Source: CAD feature listing. Evaluate the final solid. Frame: model axes, mm. Round coordinates to 2 decimals unless told otherwise and drop trailing zeros. Loops run counter-clockwise (first coordinate to the right, second up) from the corner with the lowest first, then second, coordinate; pieces in that order, holes last. Notation, with made-up numbers: (-37, 82.5) - (7, 82.5) arc R30 cw to (7, 113.5) - close; hole circle Ø1 at (29.25, 41.25). An arc over 180 degrees is marked (long way). One line per question, with ' | ' between items.
from build123d import *

# Parameters (mm, degrees)
BOSS_EXTRUDE1_DEPTH         = 6.35
FILLET1_R                   = 101.6
F_1_4_CLEARANCE_SLOT1_DEPTH = 6.35
FILLET2_R                   = 6.35


# Read off the part's stored shape, not the designer's step: 1/4 Clearance Slot1
with BuildPart() as part:
    # Sketch1 → Boss-Extrude1 (new body)
    with BuildSketch(Plane(origin=(0, 0, 0), x_dir=(0, 0, -1), z_dir=(1, 0, 0))):
        Polygon((0, 0), (0, 152.4), (654.05, 152.4), (717.55, 38.1), (717.55, 0), align=None)
    extrude(amount=BOSS_EXTRUDE1_DEPTH)

    # Fillet1
    fillet1_edges = [part.edges().sort_by_distance(p)[0] for p in [
        (3.175, 152.4, -654.05),
    ]]
    fillet(fillet1_edges, radius=FILLET1_R)

    # 1/4 Clearance Slot1 outline → 1/4 Clearance Slot1 (cut)
    with BuildSketch(Plane.YZ):
        with BuildLine():
            ThreePointArc((25.6032, -698.7032), (22.225, -695.325), (18.8468, -698.7032))
            Line((18.8468, -698.7032), (18.8468, -704.6468))
            ThreePointArc((18.8468, -704.6468), (22.225, -708.025), (25.6032, -704.6468))
            Line((25.6032, -704.6468), (25.6032, -698.7032))
        make_face()
        with BuildLine():
            Line((25.6032, -18.8468), (25.6032, -12.9032))
            ThreePointArc((25.6032, -12.9032), (22.225, -9.525), (18.8468, -12.9032))
            Line((18.8468, -12.9032), (18.8468, -18.8468))
            ThreePointArc((18.8468, -18.8468), (22.225, -22.225), (25.6032, -18.8468))
        make_face()
    extrude(amount=F_1_4_CLEARANCE_SLOT1_DEPTH, mode=Mode.SUBTRACT)

    # Fillet2
    fillet2_edges = [part.edges().sort_by_distance(p)[0] for p in [
        (3.175, 0, 0),
        (3.175, 152.4, 0),
        (3.175, 38.1, -717.55),
        (3.175, 0, -717.55),
    ]]
    fillet(fillet2_edges, radius=FILLET2_R)


solid = part.part
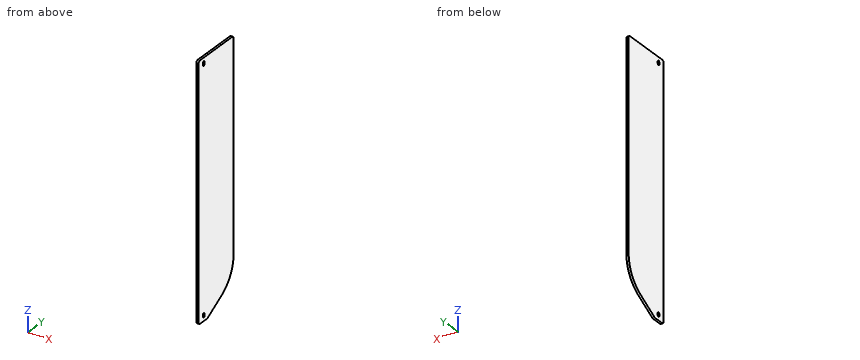
1. Section query C-C, the plane y = 86.5. Return loops of the section in (x, z), plus the area to 3 significant figures.
Worked out:
outline: (0, -690.66) - (6.35, -690.66) - (6.35, 0) - (0, 0) - close | area: 4,390 mm2
2. Contact query for a flat-ended pin moving along its axis: P1, Ø2, axis at x = 5.5, y = 110, coming from the -Z side. Output: stop coordinate, or through.
Worked out:
P1: stops at z = -677.55
3. Section query A-A, the plane x = 4.25. Return loops of the section in (y, z) (3 decimals).
Worked out:
outline: (0, -711.2) arc R6.35 ccw to (6.35, -717.55) - (36.455, -717.55) arc R6.35 ccw to (39.538, -716.751) - (100.141, -683.083) arc R101.6 ccw to (152.4, -594.268) - (152.4, -6.35) arc R6.35 ccw to (146.05, 0) - (6.35, 0) arc R6.35 ccw to (0, -6.35) - close; hole (18.847, -704.647) arc R3.378 ccw to (25.603, -704.647) - (25.603, -698.703) arc R3.378 ccw to (18.847, -698.703) - close; hole (18.847, -18.847) arc R3.378 ccw to (25.603, -18.847) - (25.603, -12.903) arc R3.378 ccw to (18.847, -12.903) - close
4. Material intervals for probe 1 along Z at (x, y) = (3.75, 24.5); probe 2 along Z at (x, y) = (4.75, 49.5); probe 3 along Z at (x, y) = (2.25, 138.5), sorted ascending.
Worked out:
probe 1: z = -717.55 to -707.14, -696.21 to -21.34, -10.41 to 0 | probe 2: z = -711.22 to 0 | probe 3: z = -645.56 to 0
5. Section query B-B, the plane y = 136. Return loops of the section in (x, z).
Worked out:
outline: (0, -649.62) - (6.35, -649.62) - (6.35, 0) - (0, 0) - close
